Design review of the part built by this model. Coordinates are the model's own, in mm. Give positions to 0.01 mm unless a question says otherwise; leave off trailing zeros. Loops run counter-clockwise (first coordinate to the right, second up) from the corner with the lowest first, then second, coordinate; pieces in that order, holes last. Notation, with made-up numbers: (-33.5, 72) -> (-11.5, 72) arc R24 cw to (-11.5, 96) -> close; hole circle Ø4 at (57, 3). An arc over 180 degrees is marked (long way). Use CSV: the item, a comma, the result in double quotes. Start each with the question number.
Item 1: We need section A-A (x = -21.59). State the section outline as (y, z) points, plus the area to 3 significant figures.
Item 2: Wall thickness on line 1 along Y through (x, z) = (-21.59, 0.2); line 2 along X through (y, z) = (2, 0.55); line 3 along X through (y, z) = (-15, 0.3): over which ranges is each line inside the solid? List them lowest first. Write a range as from..to.
Item 3: We need section C-C (z = 0.6). Count the separate pieces of the cut face and the enclosed holes in it, plus the area to 3 significant figures.
Item 4: We need section D-D (x = 24). State the section outline as (y, z) points.
Item 5: Clearance check with flat-ended pins moving along their axes: pin 1 (1.9 mm diameter, centred on x = -21.59, y = 14.29, fed in from -Z); pin 2 (1.5 mm diameter, centred on x = -19, y = -8, fed in from -Z). State where each tip first meets the part, or that it passes through.
Item 6: We need section B-B (x = -3.81). State the section outline as (y, z) points, plus the area to 3 significant figures.
from build123d import *

# Parameters (mm, degrees)
F0_R     = 1.190625
F1_DEPTH = 0.762


with BuildPart() as f1:
    # F0 (on Top) → F1 (new body)
    with BuildSketch(Plane.XY):
        with BuildLine():
            Line((-30.1625, -20.6375), (11.1125, -20.6375))
            ThreePointArc((11.1125, -20.6375), (25.705416, -14.592916), (31.75, 0))
            ThreePointArc((31.75, 0), (25.705416, 14.592916), (11.1125, 20.6375))
            Line((11.1125, 20.6375), (-30.1625, 20.6375))
            ThreePointArc((-30.1625, 20.6375), (-31.285032, 20.172532), (-31.75, 19.05))
            Line((-31.75, 19.05), (-31.75, -19.05))
            ThreePointArc((-31.75, -19.05), (-31.285032, -20.172532), (-30.1625, -20.6375))
        make_face()
        with Locations((-21.59, -14.2875)):
            Circle(F0_R, mode=Mode.SUBTRACT)
        with BuildLine():
            Line((-2.8194, 1.5494), (-2.8194, -1.5494))
            ThreePointArc((-2.8194, -1.5494), (-3.81, -2.54), (-4.8006, -1.5494))
            Line((-4.8006, -1.5494), (-4.8006, 1.5494))
            ThreePointArc((-4.8006, 1.5494), (-3.81, 2.54), (-2.8194, 1.5494))
        make_face(mode=Mode.SUBTRACT)
        with Locations((-21.59, 14.2875)):
            Circle(F0_R, mode=Mode.SUBTRACT)
    extrude(amount=F1_DEPTH)


solid = f1.part
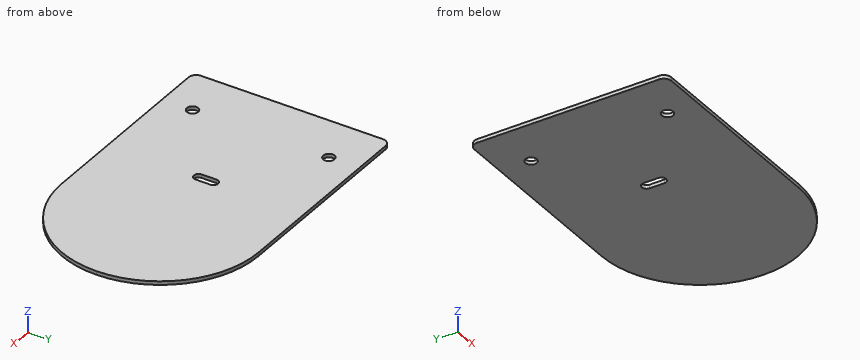
Results found:
1,outline,"(-20.64, 0) -> (-15.48, 0) -> (-15.48, 0.76) -> (-20.64, 0.76) -> close; (-13.1, 0) -> (13.1, 0) -> (13.1, 0.76) -> (-13.1, 0.76) -> close; (15.48, 0) -> (20.64, 0) -> (20.64, 0.76) -> (15.48, 0.76) -> close"
1,area,"27.8 mm²"
2,line 1,"-20.64..-15.48, -13.1..13.1, 15.48..20.64"
2,line 2,"-31.75..-4.69, -2.93..31.65"
2,line 3,"-31.75..-22.54, -20.64..25.29"
3,separate pieces,"1"
3,enclosed holes,"3"
3,area,"2,420 mm²"
4,outline,"(-16.12, 0) -> (16.12, 0) -> (16.12, 0.76) -> (-16.12, 0.76) -> close"
5,pin 1,"through"
5,pin 2,"z = 0"
6,outline,"(-20.64, 0) -> (-2.54, 0) -> (-2.54, 0.76) -> (-20.64, 0.76) -> close; (2.54, 0) -> (20.64, 0) -> (20.64, 0.76) -> (2.54, 0.76) -> close"
6,area,"27.6 mm²"
